Could you check a few things on this model? Use its own coordinates, in mm. A direction names the side the tool comes from. Round coordinates to 2 decimals unless told otherwise and drop trailing zeros. Loops run counter-clockwise (first coordinate to the right, second up) from the corner with the lowest first, then second, coordinate; pieces in that order, holes last.
Autodesk Inventor part; units mm, degrees
ref_plane "YZ Plane" through (0, 0, 0) normal (1, 0, 0) x (0, 1, 0)
ref_plane "XZ Plane" through (0, 0, 0) normal (0, 1, 0) x (-1, 0, 0)
ref_plane "XY Plane" through (0, 0, 0) normal (0, 0, 1) x (1, 0, 0)
sketch "Boceto1" plane through (0, 0, 0) normal (0, 0, 1) x (1, 0, 0)
  circle A0 centre (0, 0) radius 480
  circle A1 centre (0, 0) radius 125
  dimension "d0" = 960
  dimension "d1" = 250
extrude "Extrusión1" add sketch "Boceto1" against normal blind 25
sketch "Boceto2" plane through (0, 0, 0) normal (0, 0, 1) x (1, 0, 0)
  circle A0 centre (0, 0) radius 337
  circle A1 centre (0, 0) radius 340
  dimension "d4" = 680
  dimension "d5" = 674
extrude "Extrusión2" cut sketch "Boceto2" against normal blind 5
sketch "Boceto3" plane through (0, 0, 0) normal (0, 0, 1) x (1, 0, 0)
  arc A0 (63.1842, 356.4432) -> (-63.1842, 356.4432) centre (0, 0) ccw construction
  arc A1 (65.2787, 368.259) -> (-65.2787, 368.259) centre (0, 0) ccw
  arc A2 (61.0897, 344.6274) -> (-61.0897, 344.6274) centre (0, 0) ccw
  arc A3 (61.0897, 344.6274) -> (65.2787, 368.259) centre (63.1842, 356.4432) ccw
  arc A4 (-65.2787, 368.259) -> (-61.0897, 344.6274) centre (-63.1842, 356.4432) ccw
  line L0 (0, -74.8) -> (0, 448.8)
  point P0 (75, 354.3487)
  point P1 (-75, 354.3487)
  point P2 (0, 362)
  dimension "d8" = 12
  dimension "d9" = 362
  dimension "d15" = 150
extrude "Extrusión3" cut sketch "Boceto3" against normal up to next
properties part number "Brida_1 (flange_1) Lebus"
Item 1: If we section it at D-D, the plane y = 292: Please give me the cut outline in (x, z), then the cut area to 3 significant figures.
Results list:
outline: (-380.97, -25) - (380.97, -25) - (380.97, 0) - (174.17, 0) - (174.17, -5) - (168.24, -5) - (168.24, 0) - (-168.24, 0) - (-168.24, -5) - (-174.17, -5) - (-174.17, 0) - (-380.97, 0) - close
area: 19,000 mm2
Item 2: For faces 1 (the flat face through (-329, 77, -5)), 2 (the flat face through (100, 327, 0)), 3 (the cylindrical face through (-75.043, 354.609, -12.325)), which set-ups out of +Z, -Z, +X, -X, +Y, -Y let a thin tool reach every point of the face, with its end or its side?
Results list:
face 1: +Z
face 2: +Z, +X, -X, +Y, -Y
face 3: +Z, -Z
Item 3: If we section it at B-B, the plane x = 0: Please give me the cut outline in (y, z).
Results list:
outline: (-480, -25) - (-125, -25) - (-125, 0) - (-337, 0) - (-337, -5) - (-340, -5) - (-340, 0) - (-480, 0) - close; (125, -25) - (350, -25) - (350, 0) - (340, 0) - (340, -5) - (337, -5) - (337, 0) - (125, 0) - close; (374, -25) - (480, -25) - (480, 0) - (374, 0) - close
Item 4: If we section it at C-C, the plane z = -13.5: Please give me the cut outline in (x, y), then the cut area to 3 significant figures.
Results list:
outline: circle Ø960 at (0, 0); hole circle Ø250 at (0, 0); hole (-65.28, 368.26) arc R12 ccw to (-61.09, 344.63) arc R350 cw to (61.09, 344.63) arc R12 ccw to (65.28, 368.26) arc R374 ccw to start
area: 671,000 mm2
Item 5: Will these pins go through, and if not, where does the flat tip stop? pin 1 (1 mm diameter, centred on x = 334, z = -15.5, fed in from +Y); pin 2 (8 mm diameter, centred on y = 149, z = -12, fed in from -X); pin 3 (1.5 mm diameter, centred on y = 284, z = -22, fed in from +X).
Results list:
pin 1: stops at y = 345.22
pin 2: stops at x = -457.58
pin 3: stops at x = 387.52
Item 6: If I drill on line 1 along Y through (x, z) = (0, -2.25); line 2 along Y through (x, z) = (0, -15.5); line 3 along Y through (x, z) = (-22, -15.5), over which ranges is the centre line in solid material (lowest first)?
Results list:
line 1: y = -480 to -340, -337 to -125, 125 to 337, 340 to 350, 374 to 480
line 2: y = -480 to -125, 125 to 350, 374 to 480
line 3: y = -479.5 to -123.05, 123.05 to 349.31, 373.35 to 479.5
Item 7: We'd pull the mould along X, two halves only. Please class faces 4 (the cylindrical face through (-479.536, 21.105, -12.325)), 5 (the cylindrical face through (1, 374, -12)), 6 (the cylindrical face through (1, 350, -12)), 7 (the flat face through (100, -100, -25)): released by +X, released by -X, zero draft, split by the parting line, or undercut.
Results list:
face 4: split by the parting line
face 5: undercut
face 6: undercut
face 7: zero draft
Item 8: If we section it at A-A, the plane y = 0: Please give me the cut outline in (x, z), then the cut area to 3 significant figures.
Results list:
outline: (-480, -25) - (-125, -25) - (-125, 0) - (-337, 0) - (-337, -5) - (-340, -5) - (-340, 0) - (-480, 0) - close; (125, -25) - (480, -25) - (480, 0) - (340, 0) - (340, -5) - (337, -5) - (337, 0) - (125, 0) - close
area: 17,700 mm2
